Here's how the part is built. I have some questions about the finished solid (model axes, mm). A direction names the side the tool comes from. Give positions to 0.01 mm unless a question says otherwise; leave off trailing zeros. Order: outer loops, then holes, each group sorted by start corner. A loop starts at its lowest first (then second) coordinate and runs counter-clockwise, first axis right, second up.
from build123d import *

# Parameters (mm, degrees)
SKETCH1_W             = 100
SKETCH1_H             = 45
BOSS_EXTRUDE1_DEPTH   = 7
M3_CLEARANCE_HOLE1_D  = 3.6
M8_CLEARANCE_HOLE1_D  = 9
F_4_CLEARANCE_HOLE1_D = 3.2639
LPATTERN1_COUNT       = 4
LPATTERN1_PITCH       = 10
MIRROR1_COPY_1_D      = 3.2639
MIRROR1_COPY_2_D      = 3.2639
MIRROR1_COPY_3_D      = 3.2639
SKETCH9_W             = 7
SKETCH9_H             = 8.5
SKETCH9_W_2           = 11
CUT_EXTRUDE1_DEPTH    = 8
FILLET1_R             = 2.5


with BuildPart() as part:
    # Sketch1 → Boss-Extrude1 (new body)
    with BuildSketch(Plane(origin=(0, 0, 0), x_dir=(1, 0, 0), z_dir=(0, 1, 0))):
        Rectangle(SKETCH1_W, SKETCH1_H)
    extrude(amount=BOSS_EXTRUDE1_DEPTH)

    # M3 Clearance Hole1 (through all)
    with Locations(Plane(origin=(0, 7, 0), x_dir=(1, 0, 0), z_dir=(0, 1, 0))):
        with Locations((15.5, 15.5), (-15.5, 15.5), (-15.5, -15.5), (15.5, -15.5)):
            Hole(M3_CLEARANCE_HOLE1_D / 2)

    # M8 Clearance Hole1 (through all)
    with Locations(Plane(origin=(0, 7, 0), x_dir=(1, 0, 0), z_dir=(0, 1, 0))):
        with Locations((0, 0)):
            Hole(M8_CLEARANCE_HOLE1_D / 2)

    # #4 Clearance Hole1 (through all)
    with Locations(Plane(origin=(0, 7, 0), x_dir=(1, 0, 0), z_dir=(0, 1, 0))):
        with Locations((-42.5, 15)):
            f_4_clearance_hole1 = Hole(F_4_CLEARANCE_HOLE1_D / 2)

    # LPattern1: #4 Clearance Hole1 ×4
    with Locations(*[(0, 0, i * LPATTERN1_PITCH) for i in range(1, LPATTERN1_COUNT)]):
        add(f_4_clearance_hole1, mode=Mode.SUBTRACT)

    # Mirror1: #4 Clearance Hole1 across plane
    add(f_4_clearance_hole1.mirror(Plane(origin=(0, 0, 0), x_dir=(0, 0, 1), z_dir=(1, 0, 0))), mode=Mode.SUBTRACT)

    # Mirror1 copy 1 (through all)
    with Locations(Plane(origin=(0, 7, 10), x_dir=(-1, 0, 0), z_dir=(0, 1, 0))):
        with Locations((-42.5, -15)):
            Hole(MIRROR1_COPY_1_D / 2)

    # Mirror1 copy 2 (through all)
    with Locations(Plane(origin=(0, 7, 20), x_dir=(-1, 0, 0), z_dir=(0, 1, 0))):
        with Locations((-42.5, -15)):
            Hole(MIRROR1_COPY_2_D / 2)

    # Mirror1 copy 3 (through all)
    with Locations(Plane(origin=(0, 7, 30), x_dir=(-1, 0, 0), z_dir=(0, 1, 0))):
        with Locations((-42.5, -15)):
            Hole(MIRROR1_COPY_3_D / 2)

    # Sketch9 → Cut-Extrude1 (cut, through all)
    with BuildSketch(Plane(origin=(0, 7, 0), x_dir=(1, 0, 0), z_dir=(0, 1, 0))):
        with Locations((-29, 18.25)):
            Rectangle(SKETCH9_W, SKETCH9_H)
        with Locations((-29, -18.25)):
            Rectangle(SKETCH9_W, SKETCH9_H)
        with Locations((29, -18.25)):
            Rectangle(SKETCH9_W, SKETCH9_H)
        with Locations((29, 18.25)):
            Rectangle(SKETCH9_W, SKETCH9_H)
        with Locations((0, 18.25)):
            Rectangle(SKETCH9_W_2, SKETCH9_H)
        with Locations((0, -18.25)):
            Rectangle(SKETCH9_W_2, SKETCH9_H)
    extrude(amount=-CUT_EXTRUDE1_DEPTH, mode=Mode.SUBTRACT)

    # Fillet1
    fillet1_edges = [part.edges().sort_by_distance(p)[0] for p in [
        (5.5, 3.5, 22.5),
        (-5.5, 3.5, 22.5),
        (-5.5, 3.5, 14),
        (5.5, 3.5, 14),
        (25.5, 3.5, -22.5),
        (32.5, 3.5, -22.5),
        (32.5, 3.5, -14),
        (25.5, 3.5, -14),
        (32.5, 3.5, 22.5),
        (25.5, 3.5, 22.5),
        (25.5, 3.5, 14),
        (32.5, 3.5, 14),
        (-25.5, 3.5, 22.5),
        (-32.5, 3.5, 22.5),
        (-32.5, 3.5, 14),
        (-25.5, 3.5, 14),
        (5.5, 3.5, -22.5),
        (5.5, 3.5, -14),
        (-5.5, 3.5, -14),
        (-5.5, 3.5, -22.5),
        (-32.5, 3.5, -22.5),
        (-25.5, 3.5, -22.5),
        (-25.5, 3.5, -14),
        (-32.5, 3.5, -14),
        (-50, 3.5, -22.5),
        (50, 3.5, -22.5),
        (50, 3.5, 22.5),
        (-50, 3.5, 22.5),
    ]]
    fillet(fillet1_edges, radius=FILLET1_R)


solid = part.part
Q1. If we section it at C-C on x = 42.5: List the corners of the cut face in (y, z) for me, plus the area to 3 significant figures.
Filled sheet:
outline: (0, -22.5) - (7, -22.5) - (7, -16.63) - (0, -16.63) - close; (0, -13.37) - (7, -13.37) - (7, -6.63) - (0, -6.63) - close; (0, -3.37) - (7, -3.37) - (7, 3.37) - (0, 3.37) - close; (0, 6.63) - (7, 6.63) - (7, 13.37) - (0, 13.37) - close; (0, 16.63) - (7, 16.63) - (7, 22.5) - (0, 22.5) - close
area: 224 mm2
Q2. I need wall thicknesses on L1, parallel to Z at x = -15.5, y = 4.5; L2, parallel to Z at x = -42.5, y = 5.75; L3, parallel to X at y = 6.75, z = 19. Which ranges of each line are inside material? Lowest first, please.
Filled sheet:
L1: z = -22.5 to -17.3, -13.7 to 13.7, 17.3 to 22.5
L2: z = -22.5 to -16.63, -13.37 to -6.63, -3.37 to 3.37, 6.63 to 13.37, 16.63 to 22.5
L3: x = -50 to -32.5, -25.5 to -5.5, 5.5 to 25.5, 32.5 to 50
Q3. Thinking about a two-plate mould opening in X: for faces 1 (the face through (-49, 4, -22)), 2 (the face through (24.748, 3.451, -21.787)), 3 (the face through (-16, 3, -22.5)), which applies, released by +X, released by -X, zero draft, split by the parting line, or undercut?
Filled sheet:
face 1: released by -X
face 2: undercut
face 3: zero draft
Q4. For faces 4 (the face through (-41, 3, -22.5)), 5 (the face through (5.5, 4, 18)), 6 (the face through (32.5, 4, -18)), which set-ups out of +Z, -Z, +X, -X, +Y, -Y let a thin tool reach every point of the face, with its end or its side?
Filled sheet:
face 4: -Z, +X, -X, +Y, -Y
face 5: +Z, +Y, -Y
face 6: -Z, +Y, -Y
Q5. If we section it at B-B on x = -15.5: List the corners of the cut face in (y, z) for me.
Filled sheet:
outline: (0, -22.5) - (7, -22.5) - (7, -17.3) - (0, -17.3) - close; (0, -13.7) - (7, -13.7) - (7, 13.7) - (0, 13.7) - close; (0, 17.3) - (7, 17.3) - (7, 22.5) - (0, 22.5) - close
Q6. If we section it at D-D on x = 0: List the corners of the cut face in (y, z) for me, plus the area to 3 significant figures.
Filled sheet:
outline: (0, -14) - (7, -14) - (7, -4.5) - (0, -4.5) - close; (0, 4.5) - (7, 4.5) - (7, 14) - (0, 14) - close
area: 133 mm2
Q7. If we section it at A-A on z = 0: List the corners of the cut face in (x, y) for me.
Filled sheet:
outline: (-50, 0) - (-4.5, 0) - (-4.5, 7) - (-50, 7) - close; (4.5, 0) - (50, 0) - (50, 7) - (4.5, 7) - close
Q8. I'm going to push flat-ended pins straight in: P1, Ø2.5, axis at x = 42.5, z = 15, coming from the +Y side; P2, Ø2, axis at x = 28.5, y = 3.5, coming from the -Z side. Where does each tip first touch, or does it pass through?
Filled sheet:
P1: passes through
P2: stops at z = -14.05
